from build123d import *

# Parameters (mm, degrees)
CHAMFER1_SIZE         = 1
CHAMFER1_EDGE_2_SIZE2 = 1
CHAMFER1_EDGE_2_SIZE  = 1.162501902
SKETCH4_OUTSIDE_W     = 31.064
SKETCH4_OUTSIDE_H     = 31.064
CUT_EXTRUDE3_DEPTH    = 21.2


with BuildPart() as part:
    # Sketch1 → Revolve1 (revolve)
    with BuildSketch(Plane.XY):
        Polygon((-6.6675, 0), (-9.525, 0), (-9.525, 6), (-6.35, 6), (-6.35, 20.2), (0, 20.2), (0, -22), (-5.08, -22), (-6.6675, -10), align=None)
    revolve(axis=Axis((0, 72.046513776, 0), (0, -1, 0)))

    # Chamfer1
    chamfer1_edges = [part.edges().sort_by_distance(p)[0] for p in [
        (6.35, 20.2, 0),
    ]]
    chamfer(chamfer1_edges, length=CHAMFER1_SIZE)

    # Chamfer1 edge 2
    chamfer1_edge_2_edges = [part.edges().sort_by_distance(p)[0] for p in [
        (5.08, -22, 0),
    ]]
    chamfer(chamfer1_edge_2_edges, length=CHAMFER1_EDGE_2_SIZE, length2=CHAMFER1_EDGE_2_SIZE2)

    # Sketch4 outside → Cut-Extrude3 (cut, through all)
    with BuildSketch(Plane(origin=(0, 0, 0), x_dir=(1, 0, 0), z_dir=(0, 1, 0))):
        Rectangle(SKETCH4_OUTSIDE_W, SKETCH4_OUTSIDE_H)
        Polygon((9.814954576, 0), (4.907477288, 8.5), (-4.907477288, 8.5), (-9.814954576, 0), (-4.907477288, -8.5), (4.907477288, -8.5), align=None, mode=Mode.SUBTRACT)
    extrude(amount=CUT_EXTRUDE3_DEPTH, mode=Mode.SUBTRACT)


solid = part.part
Verification items for the finished model (mm, model axes). A direction names the side the tool comes from. Give positions to 0.01 mm unless a question says otherwise; leave off trailing zeros. Write each loop counter-clockwise with the first axis right and the second up, starting at its lowest first coordinate (ties: lowest second). Pieces come first, ordered by that corner, then holes.
(1) Access from +Z, -Z, +X, -X, +Y, -Y to the whole of each face (thin tool, end or side, straight path). Record for faces 1 (the face through (0, 3, -8.5)), 2 (the face through (0.87, -4.93, -6.61)), 3 (the face through (6.5, 6, -0.1)).
(2) Cross-section at C-C (y = -0.5). Enter the section's corners in (x, z) (1 decimal), plus the area to 3 significant figures.
(3) Cross-section at D-D (y = -15). Enter the section's corners in (x, z).
(4) Material ranges on line 1 (Z direction, x = -0.25, y = 14); line 2 (Y direction, x = 5.5, z = 4.75); line 3 (X direction, y = -18.5, z = -4.75), recorded low to high.
(5) Cross-section at A-A (x = 0). Enter the section's corners in (y, z).
(6) Gauge pin test, flat ends, axial feed: pin 1 (2 mm diameter, centred on y = -13, z = 6.5, fed in from +X); pin 2 (6 mm diameter, centred on y = -10.5, z = -4.5, fed in from -X); pin 3 (5 mm diameter, centred on x = 2.5, y = 15, fed in from -Z). Record the tip position at first contact, or that the pin passes through.
Worked out:
1. face 1: -Z, +X, -X, +Y, -Y
1. face 2: -Y
1. face 3: +Y
2. outline: circle Ø13.3 at (0, 0)
2. area: 140 mm2
3. outline: circle Ø12.01 at (0, 0)
4. line 1: z = -6.35 to 6.35
4. line 2: y = 0 to 6
4. line 3: x = -2.86 to 2.86
5. outline: (-22, -4.08) - (-20.85, -5.23) - (-10, -6.67) - (0, -6.67) - (0, -8.5) - (6, -8.5) - (6, -6.35) - (19.2, -6.35) - (20.2, -5.35) - (20.2, 5.35) - (19.2, 6.35) - (6, 6.35) - (6, 8.5) - (0, 8.5) - (0, 6.67) - (-10, 6.67) - (-20.85, 5.23) - (-22, 4.08) - close
6. pin 1: stops at x = 3.03
6. pin 2: stops at x = -6.49
6. pin 3: stops at z = -6.35
